from build123d import *

# Parameters (mm, degrees)
BOSS_EXTRUDE1_DEPTH = 10
SKETCH3_W           = 5
SKETCH3_H           = 85
BOSS_EXTRUDE2_DEPTH = 5
SKETCH5_W           = 5
SKETCH5_H           = 85
BOSS_EXTRUDE4_DEPTH = 3


with BuildPart() as part:
    # Sketch1 → Boss-Extrude1 (new body)
    with BuildSketch(Plane(origin=(0, 0, 0), x_dir=(1, 0, 0), z_dir=(0, 1, 0))):
        Polygon((0, 0), (-10, 0), (-10, -90), (-5, -90), (-5, -5), (0, -5), (5, -5), (5, 0), align=None)
    extrude(amount=BOSS_EXTRUDE1_DEPTH)

    # Sketch3 → Boss-Extrude2 (add)
    with BuildSketch(Plane(origin=(0, 10, 0), x_dir=(1, 0, 0), z_dir=(0, 1, 0))):
        with Locations((-7.5, -47.5)):
            Rectangle(SKETCH3_W, SKETCH3_H)
    extrude(amount=BOSS_EXTRUDE2_DEPTH)

    # Sketch5 → Boss-Extrude4 (add)
    with BuildSketch(Plane(origin=(0, 0, 0), x_dir=(-1, 0, 0), z_dir=(0, -1, 0))):
        with Locations((7.5, -47.5)):
            Rectangle(SKETCH5_W, SKETCH5_H)
    extrude(amount=BOSS_EXTRUDE4_DEPTH)


solid = part.part
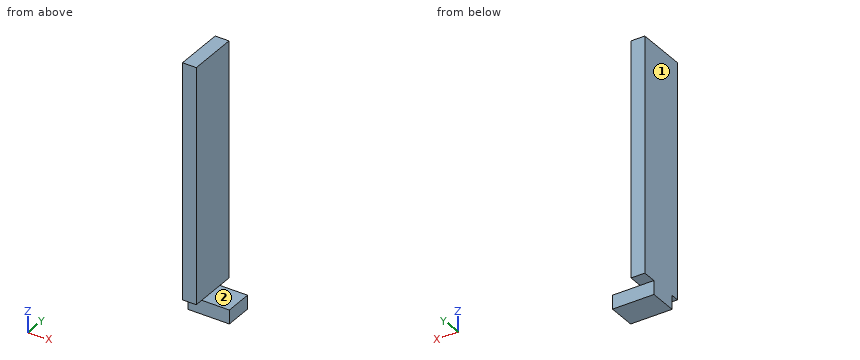
Input: part model. Units: mm. Frame: model coordinates. Face numbers are marked on the shaded views. A direction names the side the tool comes from. Round coordinates to 2 decimals unless told otherwise and drop trailing zeros. Order: outer loops, then holes, each group sorted by start corner. A loop starts at its lowest first (then second) coordinate and runs counter-clockwise, first axis right, second up.
1. Pin query (flat end, axial travel): P1, Ø6, axis at x = -2.5, y = 5.5, coming from the +Z side; P2, Ø2.5, axis at x = -3.5, z = 1.5, coming from the -Y side; P3, Ø8, axis at x = 1.5, y = 4, coming from the +Z side; P4, Ø1.5, axis at x = -7, y = 13.5, coming from the -Z side. Return the tip coordinate at first contact, or that it passes through.
The answers:
P1: stops at z = 90
P2: stops at y = 0
P3: stops at z = 5
P4: stops at z = 5
2. Cut plane D-D, the plane x = 2.25. Output: boundary loops of the cut face in (y, z).
The answers:
outline: (0, 0) - (10, 0) - (10, 5) - (0, 5) - close
3. Set-up query: the marked faces 1 and 2. Return all of +Z, -Z, +X, -X, +Y, -Y with unobstructed straight access to the full face (end or side cutting, diameter ignored); none if empty.
The answers:
face 1: +Z, -Z, -X, +Y, -Y
face 2: +Z, +X, +Y, -Y
4. Material intervals for line 1 (X direction, y = 4, z = 10.5); line 2 (Y direction, x = -3.5, z = 4); line 3 (Z direction, x = 3.25, y = 8.75), sorted ascending.
The answers:
line 1: x = -10 to -5
line 2: y = 0 to 10
line 3: z = 0 to 5
5. Cut plane B-B, the plane y = 1.5. Output: boundary loops of the cut face in (x, z).
The answers:
outline: (-10, 0) - (5, 0) - (5, 5) - (-5, 5) - (-5, 90) - (-10, 90) - close
6. Cut plane C-C, the plane z = 32. Output: boundary loops of the cut face in (x, y).
The answers:
outline: (-10, -3) - (-5, -3) - (-5, 15) - (-10, 15) - close
7. Cut plane A-A, the plane x = -8.75. Output: boundary loops of the cut face in (y, z), then the cut area to 3 significant figures.
The answers:
outline: (-3, 5) - (0, 5) - (0, 0) - (10, 0) - (10, 5) - (15, 5) - (15, 90) - (-3, 90) - close
area: 1,580 mm2
